The model under review builds one solid part; all positions refer to its coordinate system, in mm. Face numbers are marked on the shaded views. Give positions to 0.01 mm unless a question says otherwise; leave off trailing zeros. Order: outer loops, then holes, each group sorted by start corner. A loop starts at its lowest first (then second) coordinate and runs counter-clockwise, first axis right, second up. Notation, with made-up numbers: M -34,19 L -2,19 A29 cw -2,55 Z; hole C 0,14.25 d3. An arc over 180 degrees is marked long. One line per question, with ' | ' between items. Start each with the question number.
1. We need section C-C on y = 0.7. Write out the cut boundary in (x, z).
2. We need section B-B on x = 10. Write out the cut boundary in (y, z).
3. Wall thickness on L1, parallel to Z at x = 10, y = 3.2; L2, parallel to Z at x = 8, y = 5.4; L3, parallel to X at y = 1.35, z = -10: over which ranges is each line inside the solid? List them lowest first.
4. We need section D-D on x = 27.5. Write out the cut boundary in (y, z).
5. Insertion check: P1, Ø2, axis at y = 1, z = -26.5, coming from the +X side; P2, Ø5, axis at x = 10, z = -10, coming from the +Y side; P3, Ø1, axis at y = 1.5, z = -27, coming from the +X side. Each pin has a flat end and moves straight along its axis. Give the tip position at first contact, or say it passes through.
6. The part is to be moulded in two halves that separate along Z. For the marked faces 1, 2 and 3, say which applies: +Z half, -Z half, draft (parallel to the pull), parting line (faces both ways), or undercut.
7. We need section A-A on z = -10. Write out the cut boundary in (x, y), then the cut area to 3 significant figures.
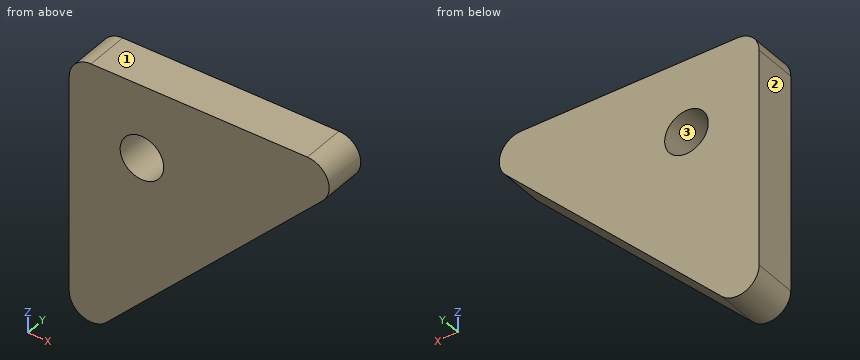
```python
from build123d import *

# Parameters (mm, degrees)
SKETCH1_R           = 3
BOSS_EXTRUDE1_DEPTH = 6


with BuildPart() as part:
    # Sketch1 → Boss-Extrude1 (new body)
    with BuildSketch(Plane(origin=(0, 0, 0), x_dir=(1, 0, 0), z_dir=(0, 1, 0))):
        with BuildLine():
            Line((5.121320344, 34.878679656), (34.878679656, 5.121320344))
            ThreePointArc((34.878679656, 5.121320344), (35.52899791, 1.851949703), (32.757359313, 0))
            Line((32.757359313, 0), (3, 0))
            ThreePointArc((3, 0), (0.878679656, 0.878679656), (0, 3))
            Line((0, 3), (0, 32.757359313))
            ThreePointArc((0, 32.757359313), (1.851949703, 35.52899791), (5.121320344, 34.878679656))
        make_face()
        with Locations((10, 10)):
            Circle(SKETCH1_R, mode=Mode.SUBTRACT)
    extrude(amount=BOSS_EXTRUDE1_DEPTH)


solid = part.part
```
Entries:
1) outline: M 0,-32.76 A3 ccw 5.12,-34.88 L 34.88,-5.12 A3 ccw 32.76,0 L 3,0 A3 ccw 0,-3 Z; hole C 10,-10 d6
2) outline: M 0,-30 L 6,-30 L 6,-13 L 0,-13 Z; M 0,-7 L 6,-7 L 6,0 L 0,0 Z
3) L1: z = -30 to -13, -7 to 0 | L2: z = -32 to -12.24, -7.76 to 0 | L3: x = 0 to 7, 13 to 30
4) outline: M 0,-12.5 L 6,-12.5 L 6,0 L 0,0 Z
5) P1: stops at x = 14.5 | P2: passes through | P3: stops at x = 13.5
6) face 1: +Z half | face 2: draft | face 3: undercut
7) outline: M 0,0 L 7,0 L 7,6 L 0,6 Z; M 13,0 L 30,0 L 30,6 L 13,6 Z | area: 144 mm^2
